Geometry: final body of the model. Coordinates: model frame, mm. A direction names the side the tool comes from. Give positions to 0.01 mm unless a question says otherwise; leave off trailing zeros. Write each loop counter-clockwise with the first axis right and the second up, starting at its lowest first coordinate (ties: lowest second). Pieces come first, ordered by that corner, then holes. Notation, with made-up numbers: M -22.75,-36 L 12.25,-36 A29 cw 12.25,-6 Z; hole C 38.5,61 d10. An arc over 180 degrees is marked long. Use one line per item in the form item = value. Start each with the question number.
Item 1: Section query D-D on y = 13. Return loops of the section in (x, z).
Item 2: Pull-direction query (X, two-part tool) for faces 3 (the flat face through (40, 20, -25)), 4 (the flat face through (15, 20, -30)), 5 (the flat face through (0, 20, -10)), 6 (the cylindrical face through (16.08, 15.12, -24.93)); classes: released by +X, released by -X, zero draft, split by the parting line, or undercut.
Item 3: Access query for faces 1 (the flat face through (39, 40, -10)), 2 (the cylindrical face through (63.92, 15.12, -24.93)). Directions: +Z, -Z, +X, -X, +Y, -Y. A direction counts if a zero-diameter tool reaches every point of the face in a straight line with its end or side. Return the directions, or none.
Item 4: Section query A-A on x = 65. Return loops of the section in (y, z), then the cut area to 3 significant figures.
Item 5: Contact query for flat-ended pins moving along their axis: P1, Ø6, axis at x = 40, y = 18.5, coming from the -Z side; P2, Ø5, axis at y = 5.5, z = -23, coming from the +X side. Output: stop coordinate, or through.
Item 6: Material intervals for line 1 along Z through (x, y) = (59, 7); line 2 along Z through (x, y) = (38.5, 27), sorted ascending. Write a range as from..to.
Item 7: Section query B-B on y = 20. Return loops of the section in (x, z).
Item 8: Section query C-C on z = -22.25. Return loops of the section in (x, y), then the cut area to 3 significant figures.
from build123d import *

# Parameters (mm, degrees)
SKETCH1_W           = 80
SKETCH1_H           = 40
BOSS_EXTRUDE1_DEPTH = 20
SKETCH2_R           = 10
BOSS_EXTRUDE2_DEPTH = 5
SKETCH3_R           = 5
BOSS_EXTRUDE3_DEPTH = 10


with BuildPart() as part:
    # Sketch1 → Boss-Extrude1 (new body)
    with BuildSketch(Plane.XY):
        with Locations((40, 20)):
            Rectangle(SKETCH1_W, SKETCH1_H)
    extrude(amount=-BOSS_EXTRUDE1_DEPTH)

    # Sketch2 → Boss-Extrude2 (add)
    with BuildSketch(Plane(origin=(0, 0, -20), x_dir=(-1, 0, 0), z_dir=(0, 0, -1))):
        with Locations((-40, 20)):
            Circle(SKETCH2_R)
    extrude(amount=BOSS_EXTRUDE2_DEPTH)

    # Sketch3 → Boss-Extrude3 (add)
    with BuildSketch(Plane(origin=(0, 0, -20), x_dir=(-1, 0, 0), z_dir=(0, 0, -1))):
        with Locations((-15, 20)):
            Circle(SKETCH3_R)
    boss_extrude3 = extrude(amount=BOSS_EXTRUDE3_DEPTH)

    # Mirror1: Boss-Extrude3 across plane
    add(boss_extrude3.mirror(Plane.ZY.offset(-40)))


solid = part.part
Answer sheet:
q1.outline = M 0,-20 L 32.86,-20 L 32.86,-25 L 47.14,-25 L 47.14,-20 L 80,-20 L 80,0 L 0,0 Z
q2.face_3 = undercut
q2.face_4 = zero draft
q2.face_5 = released by -X
q2.face_6 = undercut
q3.face_1 = +Z, -Z, +X, -X, +Y
q3.face_2 = -Z
q4.outline = M 0,-20 L 15,-20 L 15,-30 L 25,-30 L 25,-20 L 40,-20 L 40,0 L 0,0 Z
q4.area = 900 mm2
q5.P1 = -25
q5.P2 = through
q6.line_1 = -20..0
q6.line_2 = -25..0
q7.outline = M 0,-20 L 10,-20 L 10,-30 L 20,-30 L 20,-20 L 30,-20 L 30,-25 L 50,-25 L 50,-20 L 60,-20 L 60,-30 L 70,-30 L 70,-20 L 80,-20 L 80,0 L 0,0 Z
q8.outline = C 15,20 d10; C 40,20 d20; C 65,20 d10
q8.area = 471 mm2
